Model file for the job. Use its own axes, mm. A direction names the side the tool comes from. Coordinates: 2 decimals unless noted, no trailing zeros. Order: outer loops, then holes, each group sorted by start corner. A loop starts at its lowest first (then second) coordinate and runs counter-clockwise, first axis right, second up.
from build123d import *

# Parameters (mm, degrees)
SKETCH1_W           = 106.04999999
SKETCH1_H           = 50.8
BOSS_EXTRUDE1_DEPTH = 38.800000124
SKETCH3_W           = 93.34999999
SKETCH3_H           = 31.180000124
CUT_EXTRUDE1_DEPTH  = 64.516
BOSS_EXTRUDE2_DEPTH = 12.7
SKETCH8_W           = 19.05
SKETCH8_H           = 8.507235526
SKETCH8_H_2         = 8.509
BOSS_EXTRUDE3_DEPTH = 114.3
SKETCH9_W           = 19.05
SKETCH9_H           = 19.119005999
SKETCH9_H_2         = 19.115477052
BOSS_EXTRUDE4_DEPTH = 12.7
SKETCH10_W          = 8.89
SKETCH10_H          = 18.989146711
SKETCH10_H_2        = 18.987382237
BOSS_EXTRUDE5_DEPTH = 12.192
CUT_EXTRUDE7_DEPTH  = 78.232
SKETCH13_R          = 4.044043228
CUT_EXTRUDE9_DEPTH  = 83.82


with BuildPart() as part:
    # Sketch1 → Boss-Extrude1 (new body)
    with BuildSketch(Plane.XY):
        Rectangle(SKETCH1_W, SKETCH1_H)
    extrude(amount=BOSS_EXTRUDE1_DEPTH)

    # Sketch3 → Cut-Extrude1 (cut)
    with BuildSketch(Plane(origin=(0, 25.4, 0), x_dir=(1, 0, 0), z_dir=(0, 1, 0))):
        with Locations((0, -19.400000062)):
            Rectangle(SKETCH3_W, SKETCH3_H)
    extrude(amount=-CUT_EXTRUDE1_DEPTH, mode=Mode.SUBTRACT)

    # Sketch7 → Boss-Extrude2 (add)
    with BuildSketch(Plane.XY.offset(38.800000124)):
        Polygon((-37.784999995, -21.634664683), (-37.784999995, -25.4), (-18.734999995, -25.4), (-18.734999995, -21.634664683), (-18.734999995, -8.385528947), (-37.784999995, -8.385528947), align=None)
        Polygon((18.734999995, -21.634664683), (18.734999995, -25.4), (37.784999995, -25.4), (37.784999995, -21.634664683), (37.784999995, -8.382), (18.734999995, -8.382), align=None)
    extrude(amount=BOSS_EXTRUDE2_DEPTH)

    # Sketch8 → Boss-Extrude3 (add)
    with BuildSketch(Plane.XY.offset(51.500000124)):
        with Locations((-28.259999995, -21.146382237)):
            Rectangle(SKETCH8_W, SKETCH8_H)
        with Locations((28.259999995, -21.1455)):
            Rectangle(SKETCH8_W, SKETCH8_H_2)
    extrude(amount=BOSS_EXTRUDE3_DEPTH)

    # Sketch9 → Boss-Extrude4 (add)
    with BuildSketch(Plane.XY.offset(38.800000124)):
        with Locations((-28.259999995, 1.173974053)):
            Rectangle(SKETCH9_W, SKETCH9_H)
        with Locations((28.259999995, 1.175738526)):
            Rectangle(SKETCH9_W, SKETCH9_H_2)
    extrude(amount=BOSS_EXTRUDE4_DEPTH)

    # Sketch10 → Boss-Extrude5 (add)
    with BuildSketch(Plane.XY.offset(51.500000124)):
        with Locations((-28.259999995, -7.398191118)):
            Rectangle(SKETCH10_W, SKETCH10_H)
        with Locations((28.259999995, -7.397308882)):
            Rectangle(SKETCH10_W, SKETCH10_H_2)
    extrude(amount=BOSS_EXTRUDE5_DEPTH)

    # Sketch11 → Cut-Extrude7 (cut)
    with BuildSketch(Plane(origin=(32.704999995, 0, 0), x_dir=(0, 0, -1), z_dir=(1, 0, 0))):
        with BuildLine():
            ThreePointArc((-51.500000124, -16.891), (-60.993691242, -7.397308882), (-51.500000124, 2.096382237))
            Line((-51.500000124, 2.096382237), (-63.692000124, 2.096382237))
            Line((-63.692000124, 2.096382237), (-63.692000124, -16.891))
            Line((-63.692000124, -16.891), (-51.500000124, -16.891))
        make_face()
    extrude(amount=-CUT_EXTRUDE7_DEPTH, mode=Mode.SUBTRACT)

    # Sketch13 → Cut-Extrude9 (cut)
    with BuildSketch(Plane(origin=(32.704999995, 0, 0), x_dir=(0, 0, -1), z_dir=(1, 0, 0))):
        with Locations((-55.958857725, -7.397308882)):
            Circle(SKETCH13_R)
    extrude(amount=-CUT_EXTRUDE9_DEPTH, mode=Mode.SUBTRACT)


solid = part.part
Q1. Drop flat-ended pins along their axis: P1, Ø12, axis at y = 10, z = 64, coming from the +X side; P2, Ø3, axis at y = -10, z = 56, coming from the +X side (3 decimals); P3, Ø10.5, axis at y = -7.4, z = 55.96, coming from the -X side (3 decimals); P4, Ø10, axis at x = 25, z = 47.5, coming from the +Y side. Give the stop position or say it passes through.
Established:
P1: passes through
P2: stops at x = 32.705
P3: stops at x = -37.785
P4: stops at y = 10.73
Q2. Cut at A-A, the plane z = 88. List the corners of the cut face in (x, y) (3 decimals).
Established:
outline: (-37.785, -25.4) - (-18.735, -25.4) - (-18.735, -16.893) - (-37.785, -16.893) - close; (18.735, -25.4) - (37.785, -25.4) - (37.785, -16.891) - (18.735, -16.891) - close
Q3. Which spindle directions (+Z, -Z, +X, -X, +Y, -Y) get a long thin tool onto all of the face, cutting with end or side? Do faces 1 (the face through (-28, 10.733, 45)), 2 (the face through (46.675, 0, 20)), 3 (the face through (-32.705, -10, 52)). Say none if no direction does.
Established:
face 1: +Z, +X, -X, +Y
face 2: +Y, -Y
face 3: +Z, -X, +Y
Q4. Cut at C-C, the plane y = -19. List the corners of the cut face in (x, z) (3 decimals).
Established:
outline: (-53.025, 0) - (53.025, 0) - (53.025, 38.8) - (37.785, 38.8) - (37.785, 165.8) - (18.735, 165.8) - (18.735, 38.8) - (-18.735, 38.8) - (-18.735, 165.8) - (-37.785, 165.8) - (-37.785, 38.8) - (-53.025, 38.8) - close; hole (-46.675, 3.81) - (46.675, 3.81) - (46.675, 34.99) - (-46.675, 34.99) - close
Q5. Cut at B-B, the plane x = -42. List the corners of the cut face in (y, z), plus the area to 3 significant figures.
Established:
outline: (-25.4, 0) - (25.4, 0) - (25.4, 3.81) - (-25.4, 3.81) - close; (-25.4, 34.99) - (25.4, 34.99) - (25.4, 38.8) - (-25.4, 38.8) - close
area: 387 mm2
Q6. Mould opens along Y. For faces 4 (the face through (-1, 0, 0)), 5 (the face through (28.32, -7.61, 60.99)), 6 (the face through (28, 10.733, 45)), 7 (the face through (-28, -16.891, 58)) say: pulls with the +Y half, pulls with the -Y half, needs draft (parallel to the pull), parting line crosses it, or undercut.
Established:
face 4: needs draft
face 5: undercut
face 6: pulls with the +Y half
face 7: undercut
Q7. Probe line 1 (X direction, y = -7, z = 46) (3 decimals); line 2 (Z direction, x = 18.5, y = 21); line 3 (Z direction, x = -30.5, y = 8). List the from-to ranges inside material, lowest first.
Established:
line 1: x = -37.785 to -18.735, 18.735 to 37.785
line 2: z = 0 to 3.81, 34.99 to 38.8
line 3: z = 0 to 3.81, 34.99 to 51.5
Q8. Cut at D-D, the plane y = -1. List the corners of the cut face in (x, z) (3 decimals), plus the area to 3 significant figures.
Established:
outline: (-53.025, 0) - (53.025, 0) - (53.025, 38.8) - (37.785, 38.8) - (37.785, 51.5) - (32.705, 51.5) - (32.705, 58.515) - (23.815, 58.515) - (23.815, 51.5) - (18.735, 51.5) - (18.735, 38.8) - (-18.735, 38.8) - (-18.735, 51.5) - (-23.815, 51.5) - (-23.815, 58.515) - (-32.705, 58.515) - (-32.705, 51.5) - (-37.785, 51.5) - (-37.785, 38.8) - (-53.025, 38.8) - close; hole (-46.675, 3.81) - (46.675, 3.81) - (46.675, 34.99) - (-46.675, 34.99) - close
area: 1,810 mm2
